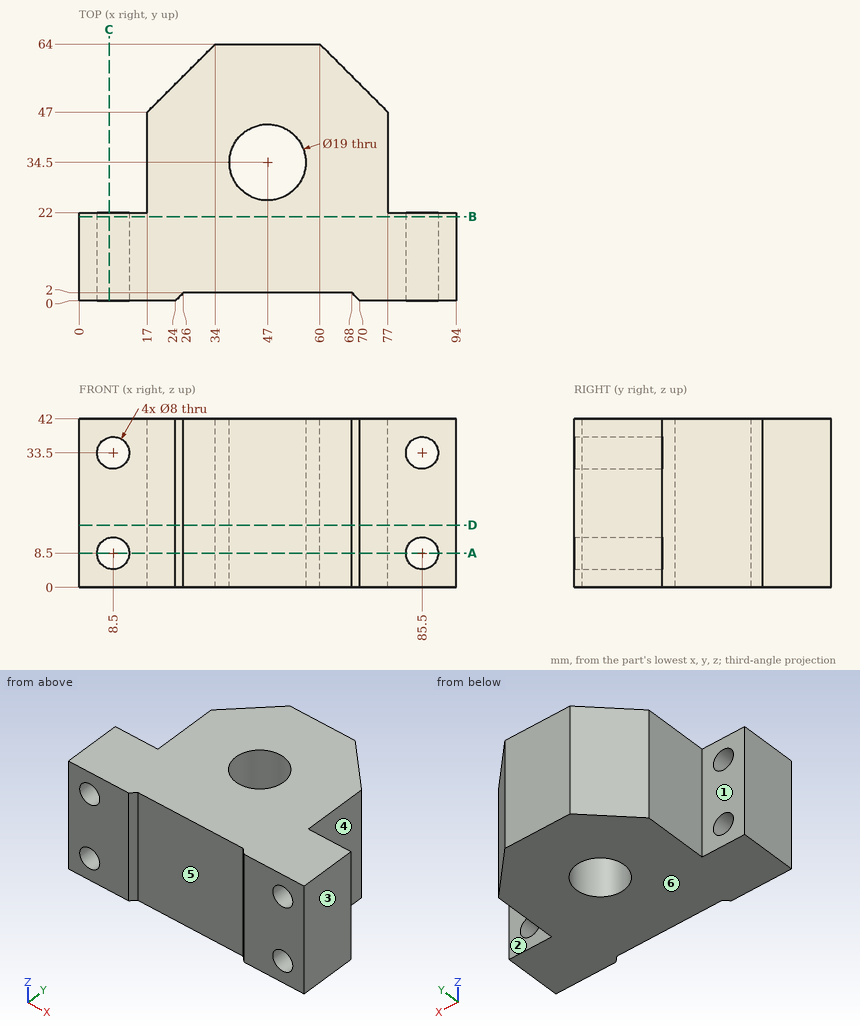
Part print with two shaded views. Sizes in mm from the minimum x, y, z corner. A direction names the side the tool comes from. Give positions to 0.01 mm unless a question says otherwise; leave off trailing zeros. Order: outer loops, then holes, each group sorted by start corner. A loop starts at its lowest first (then second) coordinate and runs counter-clockwise, first axis right, second up.
(1) Mould opens along X. For the marked faces 4, 5 and 6 say: released by +X, released by -X, zero draft, split by the parting line, or undercut.
(2) Flat gauge pins, fed straight in: pin 1 (12 mm diameter, centred on x = 54.5, z = 36, fed in from -Y); pin 2 (13.5 mm diameter, centred on x = 6.5, z = 17.5, fed in from +Y); pin 3 (12 mm diameter, centred on y = 50.5, z = 30, fed in from +X). Where does each tip first touch, or does it go through?
(3) Saw through at B-B, the plane y = 21. Give the cut face in (x, z).
(4) Tool access for the marked faces 1, 2 and 3: list every direction of +Z, -Z, +X, -X, +Y, -Y with a clear straight run to the whole face (end or side of a thin tool).
(5) Saw through at C-C, the plane x = 7.5. Give the cut face in (y, z), then the cut area to 3 significant figures.
(6) Drill centre lines: L1, parallel to X at y = 14.5, z = 8.5; L2, parallel to Y at x = 47, z = 13; L3, parallel to Z at x = 8.5, y = 13.5. Where is each one in solid material? Low to high.
(7) Saw through at D-D, the plane z = 15.5. Give the cut face in (x, y), then the cut area to 3 significant figures.
(8) Saw through at A-A, the plane z = 8.5. Give the cut face in (x, y).
Results found:
1. face 4: released by +X
1. face 5: undercut
1. face 6: zero draft
2. pin 1: stops at y = 2
2. pin 2: stops at y = 22
2. pin 3: stops at x = 77
3. outline: (0, 0) - (94, 0) - (94, 42) - (0, 42) - close; hole circle Ø8 at (8.5, 8.5); hole circle Ø8 at (8.5, 33.5); hole circle Ø8 at (85.5, 8.5); hole circle Ø8 at (85.5, 33.5)
4. face 1: +Z, -Z, -X, +Y
4. face 2: +Z, -Z, +X, +Y
4. face 3: +Z, -Z, +X, +Y, -Y
5. outline: (0, 0) - (22, 0) - (22, 4.63) - (0, 4.63) - close; (0, 12.37) - (22, 12.37) - (22, 29.63) - (0, 29.63) - close; (0, 37.37) - (22, 37.37) - (22, 42) - (0, 42) - close
5. area: 583 mm2
6. L1: x = 0 to 4.5, 12.5 to 81.5, 89.5 to 94
6. L2: y = 2 to 25, 44 to 64
6. L3: z = 0 to 4.5, 12.5 to 29.5, 37.5 to 42
7. outline: (0, 0) - (24, 0) - (26, 2) - (68, 2) - (70, 0) - (94, 0) - (94, 22) - (77, 22) - (77, 47) - (60, 64) - (34, 64) - (17, 47) - (17, 22) - (0, 22) - close; hole circle Ø19 at (47, 34.5)
7. area: 3,930 mm2
8. outline: (0, 0) - (4.5, 0) - (4.5, 22) - (0, 22) - close; (12.5, 0) - (24, 0) - (26, 2) - (68, 2) - (70, 0) - (81.5, 0) - (81.5, 22) - (77, 22) - (77, 47) - (60, 64) - (34, 64) - (17, 47) - (17, 22) - (12.5, 22) - close; (89.5, 0) - (94, 0) - (94, 22) - (89.5, 22) - close; hole circle Ø19 at (47, 34.5)
